from build123d import *

# Parameters (mm, degrees)
SKETCH1_W           = 38.275
SKETCH1_H           = 38.275
SKETCH1_R           = 15.05
BOSS_EXTRUDE1_DEPTH = 7
SKETCH2_W           = 38.275
SKETCH2_H           = 10
BOSS_EXTRUDE2_DEPTH = 45
SKETCH3_R           = 4.7
BOSS_EXTRUDE3_DEPTH = 10


with BuildPart() as part:
    # Sketch1 → Boss-Extrude1 (new body)
    with BuildSketch(Plane(origin=(0, 0, 0), x_dir=(0, 0, -1), z_dir=(1, 0, 0))):
        Rectangle(SKETCH1_W, SKETCH1_H)
        Circle(SKETCH1_R, mode=Mode.SUBTRACT)
    extrude(amount=BOSS_EXTRUDE1_DEPTH)

    # Sketch2 → Boss-Extrude2 (add)
    with BuildSketch(Plane.ZY):
        Rectangle(SKETCH2_W, SKETCH2_H)
    extrude(amount=BOSS_EXTRUDE2_DEPTH)

    # Sketch3 → Boss-Extrude3 (add)
    with BuildSketch(Plane.XY.offset(19.1375)):
        with Locations(Location((-35, 0, 0), (0, 0, 180))):
            Circle(SKETCH3_R)
        with Locations(Location((0, 0, 0), (0, 0, 180))):
            Circle(SKETCH3_R)
    boss_extrude3 = extrude(amount=BOSS_EXTRUDE3_DEPTH)

    # Mirror1: Boss-Extrude3 across plane
    add(boss_extrude3.mirror(Plane.XY))


solid = part.part
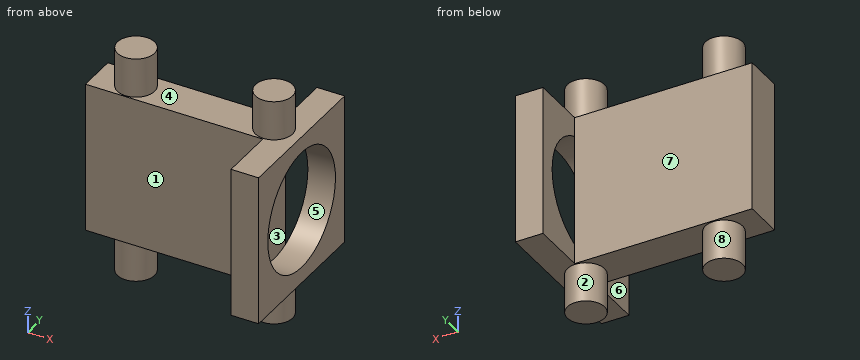
Design review of the part built by this model. Coordinates are the model's own, in mm. Face numbers are marked on the shaded views. A direction names the side the tool comes from. Coordinates: 2 decimals unless noted, no trailing zeros. Order: outer loops, then holes, each group sorted by start corner. A loop starts at its lowest first (then second) coordinate and runs counter-clockwise, first axis right, second up. Notation, with made-up numbers: (87.5, 63) -> (128.5, 63) arc R22 cw to (128.5, 82) -> close; hole circle Ø8 at (-28.5, 88.25). An arc over 180 degrees is marked (long way). Use one line per item in the form item = value. Start each with the question number.
(1) Insertion check: pin 1 (10 mm diameter, centred on x = -7, y = -2.5, fed in from +Z); pin 2 (10 mm diameter, centred on y = 13, z = 0, fed in from -X); pin 3 (1.5 mm diameter, centred on y = -0.5, z = 21.5, fed in from -X); pin 4 (19 mm diameter, centred on x = -32.5, z = -6.5, fed in from -Y). Each pin has a flat end and moves straight along its axis. Give the tip position at first contact, or say it passes through.
(2) Add section B-B on y = 0. State the section outline as (x, z) points.
(3) For the marked faces 4, 5, 6, 7 and 8, list the 3-axis set-ups (+Z, -Z, +X, -X, +Y, -Y) from which the entire face can be reached by the end or side of a thin tool; tool diameter is ignored.
(4) For probe 1 along Y at (x, z) = (3, 0); probe 2 along Z at (x, y) = (3, 0), list the stretches that pass through material, from the lowest coordinate up.
(5) The part is to be moulded in two halves that separate along Y. For the marked faces 1, 2 and 3, say which applies: +Y half, -Y half, draft (parallel to the pull), parting line (faces both ways), or undercut.
(6) Add section C-C on y = -13.5. State the section outline as (x, z) points.
(7) Add section D-D on z = -24. State the section outline as (x, y) points, plus the area to 3 significant figures.
(8) Add section A-A on z = 0. State the section outline as (x, y) points.
Answer block:
q1.pin_1 = 29.14
q1.pin_2 = 0
q1.pin_3 = -39.7
q1.pin_4 = -5
q2.outline = (-45, -19.14) -> (-39.7, -19.14) -> (-39.7, -29.14) -> (-30.3, -29.14) -> (-30.3, -19.14) -> (-4.7, -19.14) -> (-4.7, -29.14) -> (4.7, -29.14) -> (4.7, -19.14) -> (7, -19.14) -> (7, -15.05) -> (0, -15.05) -> (0, 15.05) -> (7, 15.05) -> (7, 19.14) -> (4.7, 19.14) -> (4.7, 29.14) -> (-4.7, 29.14) -> (-4.7, 19.14) -> (-30.3, 19.14) -> (-30.3, 29.14) -> (-39.7, 29.14) -> (-39.7, 19.14) -> (-45, 19.14) -> close
q3.face_4 = +Z
q3.face_5 = +X
q3.face_6 = +Z, -Z, -X, -Y
q3.face_7 = +Z, -Z, -X, +Y
q3.face_8 = -Z
q4.probe_1 = -19.14 to -15.05, 15.05 to 19.14
q4.probe_2 = -29.14 to -15.05, 15.05 to 29.14
q5.face_1 = -Y half
q5.face_2 = parting line
q5.face_3 = undercut
q6.outline = (0, -19.14) -> (7, -19.14) -> (7, -6.65) -> (0, -6.65) -> close; (0, 6.65) -> (7, 6.65) -> (7, 19.14) -> (0, 19.14) -> close
q7.outline = circle Ø9.4 at (-35, 0); circle Ø9.4 at (0, 0)
q7.area = 139 mm²
q8.outline = (-45, -5) -> (0, -5) -> (0, 5) -> (-45, 5) -> close; (0, -19.14) -> (7, -19.14) -> (7, -15.05) -> (0, -15.05) -> close; (0, 15.05) -> (7, 15.05) -> (7, 19.14) -> (0, 19.14) -> close
